```python
from build123d import *

# Parameters (mm, degrees)
SKETCH1_W                    = 380
SKETCH1_H                    = 118
BASE_FLANGE1_DEPTH           = 1.9
EDGE_FLANGE1_STRIP_W         = 9.6
EDGE_FLANGE1_STRIP_H         = 1.9
EDGE_FLANGE1_STRIP_CUT_DEPTH = 380
EDGE_FLANGE1_DEPTH           = 380
SKETCH9_R                    = 10
SKETCH9_R_2                  = 2.04
CUT_EXTRUDE1_DEPTH           = 10
SKETCH10_R                   = 2.04
CUT_EXTRUDE2_DEPTH           = 10
SKETCH11_R                   = 2.04
CUT_EXTRUDE3_DEPTH           = 10
SKETCH12_R                   = 2.04
CUT_EXTRUDE4_DEPTH           = 10
SKETCH13_R                   = 6.5
CUT_EXTRUDE5_DEPTH           = 62


# Sheet-metal steps are written as plain solids
with BuildPart() as part:
    # Sketch1 → Base-Flange1 (new body)
    with BuildSketch(Plane.XY):
        Rectangle(SKETCH1_W, SKETCH1_H)
    extrude(amount=-BASE_FLANGE1_DEPTH)

    # Edge-Flange1 strip (across the edge) → Edge-Flange1 strip cut (cut)
    with BuildSketch(Plane(origin=(190, 59, 0), x_dir=(0, -1, 0), z_dir=(-1, 0, 0))):
        with Locations((-1.9, -0.95)):
            Rectangle(EDGE_FLANGE1_STRIP_W, EDGE_FLANGE1_STRIP_H)
    extrude(amount=EDGE_FLANGE1_STRIP_CUT_DEPTH, mode=Mode.SUBTRACT)

    # Edge-Flange1 section (across the edge) → Edge-Flange1 (add)
    with BuildSketch(Plane(origin=(190, 59, 0), x_dir=(0, -1, 0), z_dir=(-1, 0, 0))):
        with BuildLine():
            Line((0, 1), (0, 13.1))
            Line((0, 13.1), (1.9, 13.1))
            Line((1.9, 13.1), (1.9, 1))
            ThreePointArc((1.9, 1), (2.192893219, 0.292893219), (2.9, 0))
            Line((2.9, 0), (2.9, -1.9))
            ThreePointArc((2.9, -1.9), (0.849390335, -1.050609665), (0, 1))
        make_face()
    extrude(amount=EDGE_FLANGE1_DEPTH)

    # Sketch9 → Cut-Extrude1 (cut)
    with BuildSketch(Plane.XY):
        with Locations((36.610673768, 30.1)):
            Circle(SKETCH9_R)
        with Locations((-128.389326232, 30.1)):
            Circle(SKETCH9_R_2)
        with Locations((111.610673768, 30.1)):
            Circle(SKETCH9_R_2)
    extrude(amount=-CUT_EXTRUDE1_DEPTH, mode=Mode.SUBTRACT)

    # Sketch10 → Cut-Extrude2 (cut)
    with BuildSketch(Plane.XZ.offset(-57.1)):
        with Locations(Location((-170, 7.52794, 0), (0, 0, 270))):
            Circle(SKETCH10_R)
        with Locations(Location((-120, 7.52794, 0), (0, 0, 270))):
            Circle(SKETCH10_R)
        with Locations(Location((170, 7.52794, 0), (0, 0, 270))):
            Circle(SKETCH10_R)
        with Locations(Location((120, 7.52794, 0), (0, 0, 270))):
            Circle(SKETCH10_R)
    extrude(amount=-CUT_EXTRUDE2_DEPTH, mode=Mode.SUBTRACT)

    # Sketch11 → Cut-Extrude3 (cut)
    with BuildSketch(Plane(origin=(0, 0, -1.9), x_dir=(-1, 0, 0), z_dir=(0, 0, -1))):
        with Locations((178.889326232, -46.1)):
            Circle(SKETCH11_R)
        with Locations((-177.652523634, -46.1)):
            Circle(SKETCH11_R)
    extrude(amount=-CUT_EXTRUDE3_DEPTH, mode=Mode.SUBTRACT)

    # Sketch12 → Cut-Extrude4 (cut)
    with BuildSketch(Plane.XY):
        with Locations((11.610673768, 41.735559355)):
            Circle(SKETCH12_R)
        with Locations((61.610673768, 41.735559355)):
            Circle(SKETCH12_R)
    extrude(amount=-CUT_EXTRUDE4_DEPTH, mode=Mode.SUBTRACT)

    # Sketch13 → Cut-Extrude5 (cut)
    with BuildSketch(Plane.XY):
        with Locations((66.610673768, 29.7737606)):
            Circle(SKETCH13_R)
    extrude(amount=-CUT_EXTRUDE5_DEPTH, mode=Mode.SUBTRACT)


solid = part.part
```
Part model, mm, in its own coordinate system. A direction names the side the tool comes from. Give positions to 0.01 mm unless a question says otherwise; leave off trailing zeros. Order: outer loops, then holes, each group sorted by start corner. A loop starts at its lowest first (then second) coordinate and runs counter-clockwise, first axis right, second up. Notation, with made-up numbers: M 62.25,25.25 L 83.25,25.25 A24 cw 83.25,42.25 Z; hole C 48.5,17.5 d8. An arc over 180 degrees is marked long. Use a Markdown table: item, result. Add a question column.
(1) Mould opens along X. For faces 3 (the face through (3, 59, 7)), 4 (the face through (61.82, 34.167, -0.937)), 5 (the face through (190, 0, -1)) say: +X half, -X half, draft (parallel to the pull), parting line (faces both ways), or undercut.
(2) Drop flat-ended pins along their axis: P1, Ø2.5, axis at x = -128.39, y = 30.1, coming from the -Z side; P2, Ø4.5, axis at x = 11.61, y = 41.74, coming from the +Z side; P3, Ø6.5, axis at x = 170, z = 7.53, coming from the -Y side. Give the stop position or say it passes through.
(3) Saw through at B-B, the plane y = -38.5. Give the cut face in (x, z), and give its area (3 significant figures).
(4) Probe line 1 along Z through (x, y) = (78, -34.5); line 2 along Y through (x, z) = (-110, 9); line 3 along Z through (x, y) = (170, 58.35). List the from-to ranges inside material, lowest first. Write a range as [from, to].
(5) Saw through at A-A, the plane x = -87.5. Give the cut face in (y, z), and give its area (4 significant figures).
(6) 3-axis set-ups, long thin cutter, end or side, ignore diameter. For faces 1 (the face through (-3, -1, 0)), 2 (the face through (-3, -1, -1.9)): which of +Z, -Z, +X, -X, +Y, -Y reach the whole face in a straight line?
Answer key:
| question | item | result |
|---|---|---|
| 1 | face 3 | draft |
| 1 | face 4 | undercut |
| 1 | face 5 | +X half |
| 2 | P1 | through |
| 2 | P2 | z = 0 |
| 2 | P3 | y = 57.1 |
| 3 | outline | M -190,-1.9 L 190,-1.9 L 190,0 L -190,0 Z |
| 3 | area | 722 mm^2 |
| 4 | line 1 | [-1.9, 0] |
| 4 | line 2 | [57.1, 59] |
| 4 | line 3 | [-0.83, 5.49], [9.57, 13.1] |
| 5 | outline | M -59,-1.9 L 56.1,-1.9 A2.9 ccw 59,1 L 59,13.1 L 57.1,13.1 L 57.1,1 A1 cw 56.1,0 L -59,0 Z |
| 5 | area | 247.5 mm^2 |
| 6 | face 1 | +Z, +X, -X, -Y |
| 6 | face 2 | -Z, +X, -X, +Y, -Y |
